Read the model definition and answer for the solid it produces. Units are mm, in the model's axes. Face numbers are marked on the shaded views. Round coordinates to 2 decimals unless told otherwise and drop trailing zeros. Order: outer loops, then holes, each group sorted by start corner. A loop starts at its lowest first (then second) coordinate and runs counter-clockwise, first axis right, second up. Notation, with made-up numbers: (-38.5, 69) -> (4.5, 69) arc R18 cw to (4.5, 98) -> close; hole circle Ø5 at (7.5, 18). An arc over 180 degrees is marked (long way). Answer as a JSON object with one key per item and string values. Group by question number.
Item 1: Consider probe 1 along Y at (x, z) = (0, 8.4); probe 2 along Z at (x, y) = (-0.25, 3.25); probe 3 along Z at (x, y) = (0.5, 0). Determine where each line is inside the solid, lowest interval first. Write a range as from..to.
Item 2: Section C-C, the plane z = 1.5 is taken. Write down the section's boundary in (x, y), plus the area to 3 significant figures.
Item 3: Section A-A, the plane x = 0 is taken. Write down the section's boundary in (y, z), plus the area to 3 significant figures.
Item 4: The mould has two halves that part along Y. Classify the marked faces 1, 2 and 3: pulls with the +Y half, pulls with the -Y half, needs draft (parallel to the pull), parting line crosses it, or undercut.
Item 5: Given P1, Ø1, axis at x = 0.5, y = 2.5, coming from the -Z side; P2, Ø1, axis at x = 3, y = 2.5, coming from the +Z side, each flat-ended and moving along its own axis, determine where each tip first touches the part or whether it passes through.
Item 6: Section D-D, the plane y = 2.5 is taken. Write down the section's boundary in (x, z), plus the area to 3 significant figures.
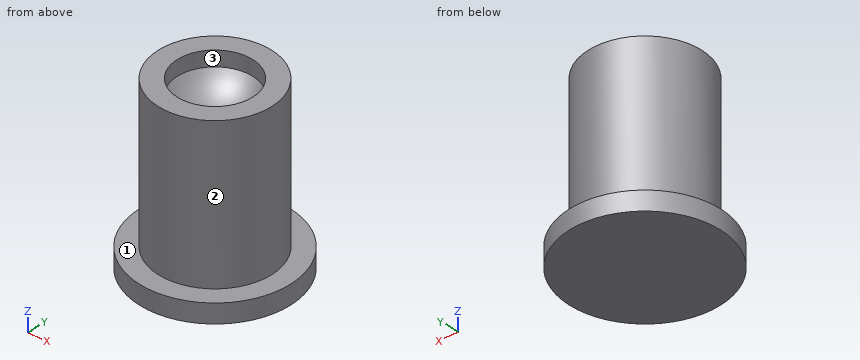
from build123d import *

# Parameters (mm, degrees)
SKETCH2_R           = 4
BOSS_EXTRUDE1_DEPTH = 1
SKETCH3_R           = 3
BOSS_EXTRUDE2_DEPTH = 8
SKETCH4_R           = 2
CUT_EXTRUDE4_DEPTH  = 0.8
DOME2_FACE_RADIUS   = 2
DOME2_HEIGHT        = 1


with BuildPart() as part:
    # Sketch2 → Boss-Extrude1 (new body)
    with BuildSketch(Plane.XY):
        Circle(SKETCH2_R)
    extrude(amount=BOSS_EXTRUDE1_DEPTH)

    # Sketch3 → Boss-Extrude2 (add)
    with BuildSketch(Plane.XY.offset(1)):
        Circle(SKETCH3_R)
    extrude(amount=BOSS_EXTRUDE2_DEPTH)

    # Sketch4 → Cut-Extrude4 (cut)
    with BuildSketch(Plane.XY.offset(9)):
        Circle(SKETCH4_R)
    extrude(amount=-CUT_EXTRUDE4_DEPTH, mode=Mode.SUBTRACT)

    # Dome2: a dome of height H over a round flat face of radius A is a cap of a sphere of radius (A * A + H * H) / (2 * H)
    dome2_r = (DOME2_FACE_RADIUS * DOME2_FACE_RADIUS + DOME2_HEIGHT * DOME2_HEIGHT) / (2 * DOME2_HEIGHT)
    dome2_base = Plane((0, 0, 8.2), z_dir=(0, 0, -1))
    with Locations(dome2_base.offset(DOME2_HEIGHT - dome2_r)):
        dome2_ball = Sphere(dome2_r, mode=Mode.PRIVATE)
    add(split(dome2_ball, bisect_by=dome2_base, keep=Keep.TOP, mode=Mode.PRIVATE), mode=Mode.SUBTRACT)


solid = part.part
Values found:
{
 "1": {"probe 1": "-3..-2, 2..3", "probe 2": "0..1", "probe 3": "0..7.25"},
 "2": {"outline": "circle Ø6 at (0, 0)", "area": "28.3 mm2"},
 "3": {"outline": "(-4, 0) -> (4, 0) -> (4, 1) -> (3, 1) -> (3, 9) -> (2, 9) -> (2, 8.2) arc R2.5 cw to (-2, 8.2) -> (-2, 9) -> (-3, 9) -> (-3, 1) -> (-4, 1) -> close", "area": "50.0 mm2"},
 "4": {"face 1": "needs draft", "face 2": "parting line crosses it", "face 3": "undercut"},
 "5": {"P1": "z = 0", "P2": "z = 1"},
 "6": {"outline": "(-3.12, 0) -> (3.12, 0) -> (3.12, 1) -> (1.66, 1) -> (1.66, 9) -> (-1.66, 9) -> (-1.66, 1) -> (-3.12, 1) -> close", "area": "32.8 mm2"}
}
